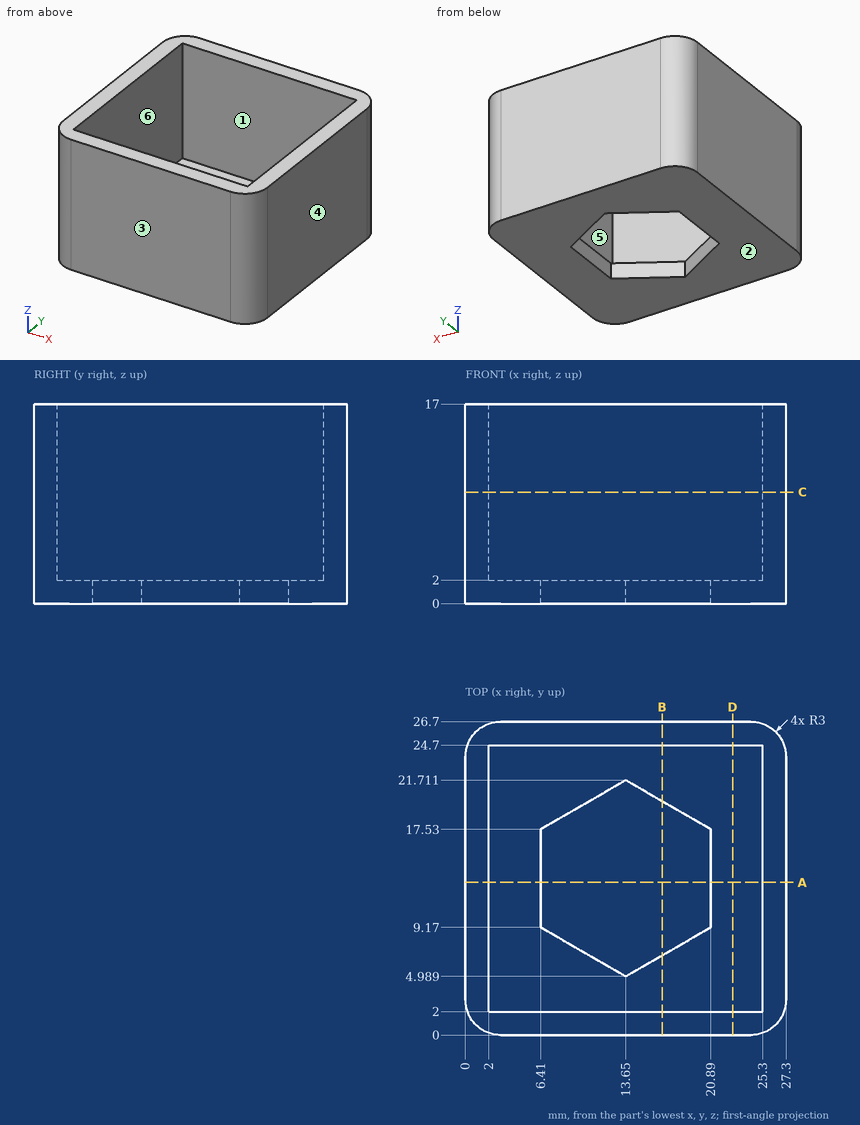
Job drawing, mm, ordinate dimensions from the low corner. One solid piece. A direction names the side the tool comes from. Give positions to 0.01 mm unless a question says otherwise; leave off trailing zeros. Loops run counter-clockwise (first coordinate to the right, second up) from the corner with the lowest first, then second, coordinate; pieces in that order, holes last. Notation, with made-up numbers: M -22,86 L 21,86 A13 ccw 21,102 Z; hole C -22.75,78.5 d8. An arc over 180 degrees is marked long. Put each result on its own line as item: value. Start each with the question number.
1) Saw through at B-B (x = 16.75). List the corners of the cut face in (y, z).
2) Flat gauge pin, fed straight in: pin 1 (7 mm diameter, centred on x = 17, y = 9, fed in from +Z). Where does the tip first touch, or does it go through?
3) Saw through at A-A (y = 13). List the corners of the cut face in (x, z).
4) 3-axis set-ups, long thin cutter, end or side, ignore diameter. For the marked faces 1 and 2: which of +Z, -Z, +X, -X, +Y, -Y reach the whole face in a straight line?
5) Probe probe 1 along X at (y, z) = (4.25, 7); probe 2 along Y at (x, z) = (19, 15.5); probe 3 along Z at (x, y) = (8.5, 2.25). List the from-to ranges inside material, lowest first.
6) Saw through at C-C (z = 9.5). List the corners of the cut face in (x, y).
7) Pull direction Y, two halves, no side cores. Call the marked faces 3, 4, 5 and 6: +Y half, -Y half, draft (parallel to the pull), parting line (faces both ways), or undercut.
8) Saw through at D-D (x = 22.75). List the corners of the cut face in (y, z).
Numbers:
1. outline: M 0,0 L 6.78,0 L 6.78,2 L 2,2 L 2,17 L 0,17 Z; M 19.92,0 L 26.7,0 L 26.7,17 L 24.7,17 L 24.7,2 L 19.92,2 Z
2. pin 1: z = 2
3. outline: M 0,0 L 6.41,0 L 6.41,2 L 2,2 L 2,17 L 0,17 Z; M 20.89,0 L 27.3,0 L 27.3,17 L 25.3,17 L 25.3,2 L 20.89,2 Z
4. face 1: +Z
4. face 2: -Z, +X, -X, +Y, -Y
5. probe 1: 0 to 2, 25.3 to 27.3
5. probe 2: 0 to 2, 24.7 to 26.7
5. probe 3: 0 to 2
6. outline: M 0,3 A3 ccw 3,0 L 24.3,0 A3 ccw 27.3,3 L 27.3,23.7 A3 ccw 24.3,26.7 L 3,26.7 A3 ccw 0,23.7 Z; hole M 2,2 L 25.3,2 L 25.3,24.7 L 2,24.7 Z
7. face 3: -Y half
7. face 4: draft
7. face 5: undercut
7. face 6: undercut
8. outline: M 0,0 L 26.7,0 L 26.7,17 L 24.7,17 L 24.7,2 L 2,2 L 2,17 L 0,17 Z
